from build123d import *

# Parameters (mm, degrees)
ESQUISSE1_W             = 37
ESQUISSE1_H             = 54
BOSS_EXTRU_1_DEPTH      = 20
BOSS_EXTRU_2_DEPTH      = 2
ESQUISSE3_W             = 6
ESQUISSE3_H             = 7
ENL_V_MAT_EXTRU_1_DEPTH = 52.478150705
ESQUISSE4_W             = 6
ESQUISSE4_H             = 7
ENL_V_MAT_EXTRU_2_DEPTH = 52.478150705
BOSS_EXTRU_3_DEPTH      = 2
ESQUISSE6_W             = 28.6
ESQUISSE6_H             = 6.8
ENL_V_MAT_EXTRU_3_DEPTH = 52.478150705
ENL_V_MAT_EXTRU_4_DEPTH = 41.582754958
ENL_V_MAT_EXTRU_5_DEPTH = 41.582754958
ESQUISSE9_W             = 28.6
ESQUISSE9_H             = 6.8
ENL_V_MAT_EXTRU_6_DEPTH = 52.478150705
ENL_V_MAT_EXTRU_7_DEPTH = 43.308391603
ENL_V_MAT_EXTRU_8_DEPTH = 43.308391603
ESQUISSE12_W            = 2.05
ESQUISSE12_H            = 2.4
ESQUISSE13_W            = 2.05
ESQUISSE13_H            = 2.4
ESQUISSE14_W            = 2.05
ESQUISSE14_H            = 2.4
ESQUISSE15_W            = 2.05
ESQUISSE15_H            = 2.4


with BuildPart() as part:
    # Esquisse1 → Boss.-Extru.1 (new body)
    with BuildSketch(Plane(origin=(10, 0, 0), x_dir=(0, 0, -1), z_dir=(1, 0, 0))):
        with Locations((-18.5, 0)):
            Rectangle(ESQUISSE1_W, ESQUISSE1_H)
    extrude(amount=-BOSS_EXTRU_1_DEPTH)

    # Esquisse2 → Boss.-Extru.2 (add)
    with BuildSketch(Plane.XY.offset(37)):
        with BuildLine():
            Line((-9, -14), (-9, 5.641101056))
            ThreePointArc((-9, 5.641101056), (0, 20), (9, 5.641101056))
            Line((9, 5.641101056), (9, -14))
            Line((9, -14), (-9, -14))
        make_face()
    extrude(amount=BOSS_EXTRU_2_DEPTH)

    # Esquisse3 → Enlèv. mat.-Extru.1 (cut, through all)
    with BuildSketch(Plane(origin=(10, 0, 0), x_dir=(0, 0, -1), z_dir=(1, 0, 0))):
        with Locations((-34, 23.5)):
            Rectangle(ESQUISSE3_W, ESQUISSE3_H)
    extrude(amount=-ENL_V_MAT_EXTRU_1_DEPTH, mode=Mode.SUBTRACT)

    # Esquisse4 → Enlèv. mat.-Extru.2 (cut, through all)
    with BuildSketch(Plane.ZY.offset(10)):
        with Locations((34, -23.5)):
            Rectangle(ESQUISSE4_W, ESQUISSE4_H)
    extrude(amount=-ENL_V_MAT_EXTRU_2_DEPTH, mode=Mode.SUBTRACT)

    # Esquisse5 → Boss.-Extru.3 (add)
    with BuildSketch(Plane.XY.offset(37)):
        with BuildLine():
            Line((-5, -14), (5, -14))
            ThreePointArc((5, -14), (0, -16), (-5, -14))
        make_face()
    extrude(amount=BOSS_EXTRU_3_DEPTH)

    # Esquisse6 → Enlèv. mat.-Extru.3 (cut, through all)
    with BuildSketch(Plane.ZY.offset(10)):
        with Locations((14.3, -23.6)):
            Rectangle(ESQUISSE6_W, ESQUISSE6_H)
    extrude(amount=-ENL_V_MAT_EXTRU_3_DEPTH, mode=Mode.SUBTRACT)

    # Esquisse7 → Enlèv. mat.-Extru.4 (cut, through all)
    with BuildSketch(Plane(origin=(0, 0, 28.6), x_dir=(-1, 0, 0), z_dir=(0, 0, -1))):
        with BuildLine():
            Line((3.75, -27), (6.25, -27))
            Line((6.25, -27), (6.25, -25.124807681))
            ThreePointArc((6.25, -25.124807681), (5, -25.55), (3.75, -25.124807681))
            Line((3.75, -25.124807681), (3.75, -27))
        make_face()
    extrude(amount=-ENL_V_MAT_EXTRU_4_DEPTH, mode=Mode.SUBTRACT)

    # Esquisse8 → Enlèv. mat.-Extru.5 (cut, through all)
    with BuildSketch(Plane(origin=(0, 0, 28.6), x_dir=(-1, 0, 0), z_dir=(0, 0, -1))):
        with BuildLine():
            Line((-6.25, -27), (-3.75, -27))
            Line((-3.75, -27), (-3.75, -25.124807681))
            ThreePointArc((-3.75, -25.124807681), (-5, -25.55), (-6.25, -25.124807681))
            Line((-6.25, -25.124807681), (-6.25, -27))
        make_face()
    extrude(amount=-ENL_V_MAT_EXTRU_5_DEPTH, mode=Mode.SUBTRACT)

    # Esquisse9 → Enlèv. mat.-Extru.6 (cut, through all)
    with BuildSketch(Plane.ZY.offset(10)):
        with Locations((14.3, 23.6)):
            Rectangle(ESQUISSE9_W, ESQUISSE9_H)
    extrude(amount=-ENL_V_MAT_EXTRU_6_DEPTH, mode=Mode.SUBTRACT)

    # Esquisse10 → Enlèv. mat.-Extru.7 (cut, through all)
    with BuildSketch(Plane.XY.offset(31)):
        with BuildLine():
            Line((-3.75, 27), (-6.25, 27))
            Line((-6.25, 27), (-6.25, 25.124807681))
            ThreePointArc((-6.25, 25.124807681), (-5, 25.55), (-3.75, 25.124807681))
            Line((-3.75, 25.124807681), (-3.75, 27))
        make_face()
    extrude(amount=-ENL_V_MAT_EXTRU_7_DEPTH, mode=Mode.SUBTRACT)

    # Esquisse11 → Enlèv. mat.-Extru.8 (cut, through all)
    with BuildSketch(Plane.XY.offset(31)):
        with BuildLine():
            Line((6.25, 27), (3.75, 27))
            Line((3.75, 27), (3.75, 25.124807681))
            ThreePointArc((3.75, 25.124807681), (5, 25.55), (6.25, 25.124807681))
            Line((6.25, 25.124807681), (6.25, 27))
        make_face()
    extrude(amount=-ENL_V_MAT_EXTRU_8_DEPTH, mode=Mode.SUBTRACT)

    # Esquisse12 → Enlèvement de matière-Révolution1 (revolve, cut)
    with BuildSketch(Plane(origin=(0, 23.5, 0), x_dir=(1, 0, 0), z_dir=(0, 1, 0))):
        with Locations((6.025, -29.8)):
            Rectangle(ESQUISSE12_W, ESQUISSE12_H)
    revolve(axis=Axis((5, 23.5, 28.6), (0, 0, 1)), mode=Mode.SUBTRACT)

    # Esquisse13 → Enlèvement de matière-Révolution2 (revolve, cut)
    with BuildSketch(Plane.XZ.offset(-23.5)):
        with Locations((-3.975, 29.8)):
            Rectangle(ESQUISSE13_W, ESQUISSE13_H)
    revolve(axis=Axis((-5, 23.5, 31), (0, 0, -1)), mode=Mode.SUBTRACT)

    # Esquisse14 → Enlèvement de matière-Révolution3 (revolve, cut)
    with BuildSketch(Plane(origin=(0, -23.5, 0), x_dir=(1, 0, 0), z_dir=(0, 1, 0))):
        with Locations((-3.975, -29.8)):
            Rectangle(ESQUISSE14_W, ESQUISSE14_H)
    revolve(axis=Axis((-5, -23.5, 28.6), (0, 0, 1)), mode=Mode.SUBTRACT)

    # Esquisse15 → Enlèvement de matière-Révolution4 (revolve, cut)
    with BuildSketch(Plane.XZ.offset(23.5)):
        with Locations((6.025, 29.8)):
            Rectangle(ESQUISSE15_W, ESQUISSE15_H)
    revolve(axis=Axis((5, -23.5, 31), (0, 0, -1)), mode=Mode.SUBTRACT)

    # Esquisse16 → Révolution1 (revolve)
    with BuildSketch(Plane.XZ.offset(-10), mode=Mode.PRIVATE) as r_volution1_sk:
        Polygon((3, 45.3), (0, 45.3), (0, 39), (6.5, 39), (6.5, 40.3), (5.35, 40.3), (5.35, 40.8), (3, 40.8), align=None)
    revolve(r_volution1_sk.sketch.rotate(Axis((0, 10, 45.3), (0, 0, -1)), 180), axis=Axis((0, 10, 45.3), (0, 0, -1)))


solid = part.part
Geometry check sheet. Reference: the model listing, model coordinates, mm. A direction names the side the tool comes from. Give positions to 0.01 mm unless a question says otherwise; leave off trailing zeros. Loops run counter-clockwise (first coordinate to the right, second up) from the corner with the lowest first, then second, coordinate; pieces in that order, holes last. Notation, with made-up numbers: M 75,86.25 L 123,86.25 A23 cw 123,95.25 Z; hole C 54.25,59 d5. An arc over 180 degrees is marked long. Write each question's results on one line, items separated by ' | '.
1) Section check C-C, the plane z = 33.5. Record the boundary of the cut face in (x, y), plus the area to 3 significant figures.
Answers follow:
outline: M -10,-20 L 10,-20 L 10,20 L -10,20 Z | area: 800 mm2
2) Section check D-D, the plane y = 18. Record the boundary of the cut face in (x, z), plus the area to 3 significant figures.
Answers follow:
outline: M -10,0 L 10,0 L 10,37 L 6,37 L 6,39 L -6,39 L -6,37 L -10,37 Z | area: 764 mm2
3) Release check for a two-part mould opening along Y. For faces 5 (the face through (0, 23, 31)), 6 (the face through (-4.93, 21.45, 29.82)), 7 (the face through (0, 20, 34)) record: +Y half, -Y half, draft (parallel to the pull), parting line (faces both ways), or undercut.
Answers follow:
face 5: draft | face 6: undercut | face 7: +Y half
4) Thickness scan on line 1 (X direction, y = -23.5, z = 30.35); line 2 (Y direction, x = 1.25, z = 23); line 3 (X direction, y = -1, z = 38). Record the ranges inside material, lowest first.
Answers follow:
line 1: -10 to -7.05, -2.95 to 2.95, 7.05 to 10 | line 2: -20.2 to 20.2 | line 3: -9 to 9
5) Gauge pin test, flat ends, axial feed: pin 1 (1.6 mm diameter, centred on y = -4.5, z = 38, fed in from -X); pin 2 (7.5 mm diameter, centred on x = -4.5, y = -24.5, fed in from +Z); pin 3 (6 mm diameter, centred on x = -1, z = 11, fed in from -Y). Record the tip position at first contact, or that the pin passes through.
Answers follow:
pin 1: x = -9 | pin 2: z = 31 | pin 3: y = -20.2
6) Section check A-A, the plane y = 23.5. Record the boundary of the cut face in (x, z), plus the area to 3 significant figures.
Answers follow:
outline: M -10,28.6 L -7.05,28.6 L -7.05,31 L -10,31 Z; M -2.95,28.6 L 2.95,28.6 L 2.95,31 L -2.95,31 Z; M 7.05,28.6 L 10,28.6 L 10,31 L 7.05,31 Z | area: 28.3 mm2
7) Tool access check on faces 1 (the face through (1.16, 4.777, 40.554)), 2 (the face through (0, -20.2, 14)), 3 (the face through (3.75, -26, 30)), 4 (the face through (0, -24, 31)). Record the directions out of +Z, -Z, +X, -X, +Y, -Y that give a thin tool (end or side, any length) a straight path to the whole face; none if there is none.
Answers follow:
face 1: +Z | face 2: -Z, +X, -X, -Y | face 3: +Z, -Z, -Y | face 4: +Z, +X, -X, -Y
8) Section check B-B, the plane y = 0.5. Record the boundary of the cut face in (x, z).
Answers follow:
outline: M -10,0 L 10,0 L 10,37 L 9,37 L 9,39 L -9,39 L -9,37 L -10,37 Z
